```python
from build123d import *

# Parameters (mm, degrees)
SKETCH1_W           = 30
SKETCH1_H           = 70
BOSS_EXTRUDE1_DEPTH = 10.5
SKETCH2_W           = 30
SKETCH2_H           = 35
CUT_EXTRUDE1_DEPTH  = 8
SKETCH3_R           = 3.1
CUT_EXTRUDE2_DEPTH  = 48.2784306
SKETCH4_R           = 1.6
CUT_EXTRUDE3_DEPTH  = 40.5
SKETCH5_W           = 7
SKETCH5_H           = 7
BOSS_EXTRUDE2_DEPTH = 4.5
CUT_EXTRUDE4_REACH  = 76.123
SKETCH6_R           = 1.6


with BuildPart() as part:
    # Sketch1 → Boss-Extrude1 (new body)
    with BuildSketch(Plane(origin=(0, 0, 0), x_dir=(1, 0, 0), z_dir=(0, 1, 0))):
        Rectangle(SKETCH1_W, SKETCH1_H)
    extrude(amount=BOSS_EXTRUDE1_DEPTH)

    # Sketch2 → Cut-Extrude1 (cut)
    with BuildSketch(Plane(origin=(0, 10.5, 0), x_dir=(1, 0, 0), z_dir=(0, 1, 0))):
        Rectangle(SKETCH2_W, SKETCH2_H)
    extrude(amount=-CUT_EXTRUDE1_DEPTH, mode=Mode.SUBTRACT)

    # Sketch3 → Cut-Extrude2 (cut, through all)
    with BuildSketch(Plane(origin=(15, 0, 0), x_dir=(0, 0, -1), z_dir=(1, 0, 0))):
        with Locations((-23, 11.5)):
            Circle(SKETCH3_R)
        with Locations((23, 11.5)):
            Circle(SKETCH3_R)
    extrude(amount=-CUT_EXTRUDE2_DEPTH, mode=Mode.SUBTRACT)

    # Sketch4 → Cut-Extrude3 (cut, through all)
    with BuildSketch(Plane(origin=(0, 10.5, 0), x_dir=(1, 0, 0), z_dir=(0, 1, 0))):
        with Locations(Location((-9.5, -31.5, 0), (0, 0, 270))):
            Circle(SKETCH4_R)
        with Locations(Location((9.5, -31.5, 0), (0, 0, 270))):
            Circle(SKETCH4_R)
        with Locations(Location((-9.5, 28.75, 0), (0, 0, 270))):
            Circle(SKETCH4_R)
        with Locations(Location((9.5, 28.75, 0), (0, 0, 270))):
            Circle(SKETCH4_R)
    extrude(amount=-CUT_EXTRUDE3_DEPTH, mode=Mode.SUBTRACT)

    # Sketch5 → Boss-Extrude2 (add)
    with BuildSketch(Plane(origin=(0, 0, -35), x_dir=(-1, 0, 0), z_dir=(0, 0, -1))):
        with Locations((18.5, 7)):
            Rectangle(SKETCH5_W, SKETCH5_H)
        with Locations((-18.5, 7)):
            Rectangle(SKETCH5_W, SKETCH5_H)
    extrude(amount=-BOSS_EXTRUDE2_DEPTH)

    # Sketch6 → Cut-Extrude4 (cut, up to next)
    with BuildSketch(Plane(origin=(0, 0, -35), x_dir=(-1, 0, 0), z_dir=(0, 0, -1)), mode=Mode.PRIVATE) as cut_extrude4_sk1:
        with Locations((-18.5, 7)):
            Circle(SKETCH6_R)
    cut_extrude4_tool1 = extrude(cut_extrude4_sk1.sketch, amount=-CUT_EXTRUDE4_REACH, mode=Mode.PRIVATE) & part.part
    # Sketch6 → Cut-Extrude4 (cut, up to next)
    with BuildSketch(Plane(origin=(0, 0, -35), x_dir=(-1, 0, 0), z_dir=(0, 0, -1)), mode=Mode.PRIVATE) as cut_extrude4_sk2:
        with Locations((18.5, 7)):
            Circle(SKETCH6_R)
    cut_extrude4_tool2 = extrude(cut_extrude4_sk2.sketch, amount=-CUT_EXTRUDE4_REACH, mode=Mode.PRIVATE) & part.part
    add(cut_extrude4_tool1.solids().sort_by_distance((18.5, 7, -35))[0], mode=Mode.SUBTRACT)
    add(cut_extrude4_tool2.solids().sort_by_distance((-18.5, 7, -35))[0], mode=Mode.SUBTRACT)


solid = part.part
```
Could you check a few things on this model? Use its own coordinates, in mm. A direction names the side the tool comes from. Coordinates: 2 decimals unless noted, no trailing zeros. Loops run counter-clockwise (first coordinate to the right, second up) from the corner with the lowest first, then second, coordinate; pieces in that order, holes last.
1) Imagine slicing it at A-A (x = -18.5). List the corners of the cut face in (y, z) for me, and give its area (3 significant figures).
Reported:
outline: (3.5, -35) - (5.4, -35) - (5.4, -30.5) - (3.5, -30.5) - close; (8.6, -35) - (10.5, -35) - (10.5, -30.5) - (8.6, -30.5) - close
area: 17.1 mm2
2) Please list where these lines run through material, in increasing order: line 1 along X through (y, z) = (2.5, -28.75); line 2 along Y through (x, z) = (-18.5, -32.5); line 3 along Z through (x, y) = (-2, 8).
Reported:
line 1: x = -15 to -11.1, -7.9 to 7.9, 11.1 to 15
line 2: y = 3.5 to 5.4, 8.6 to 10.5
line 3: z = -35 to -17.5, 17.5 to 35
3) Imagine slicing it at B-B (y = 7). List the corners of the cut face in (x, z) for me, and give its area (3 significant figures).
Reported:
outline: (-22, -35) - (-20.1, -35) - (-20.1, -30.5) - (-22, -30.5) - close; (-16.9, -35) - (16.9, -35) - (16.9, -30.5) - (15, -30.5) - (15, -17.5) - (-15, -17.5) - (-15, -30.5) - (-16.9, -30.5) - close; (-15, 17.5) - (15, 17.5) - (15, 35) - (-15, 35) - close; (20.1, -35) - (22, -35) - (22, -30.5) - (20.1, -30.5) - close; hole circle Ø3.2 at (-9.5, -28.75); hole circle Ø3.2 at (-9.5, 31.5); hole circle Ø3.2 at (9.5, -28.75); hole circle Ø3.2 at (9.5, 31.5)
area: 1,050 mm2
4) Imagine slicing it at D-D (y = 1). List the corners of the cut face in (x, z) for me.
Reported:
outline: (-15, -35) - (15, -35) - (15, 35) - (-15, 35) - close; hole circle Ø3.2 at (-9.5, -28.75); hole circle Ø3.2 at (-9.5, 31.5); hole circle Ø3.2 at (9.5, -28.75); hole circle Ø3.2 at (9.5, 31.5)
5) Will these pins go through, and if not, where does the flat tip stop? pin 1 Ø1.3 at (x, z) = (-18, -32) entering from -Y; pin 2 Ø5.5 at (x, y) = (-17, 6) entering from +Z; pin 3 Ø1.9 at (x, z) = (-9.5, 31.5) entering from +Y; pin 4 Ø5 at (y, z) = (9.5, -16) entering from +X.
Reported:
pin 1: stops at y = 3.5
pin 2: stops at z = 35
pin 3: passes through
pin 4: stops at x = 15
6) Which directions (+Z, -Z, +X, -X, +Y, -Y) give clear straight access to the entire face, cutting with the end or side of a thin tool? Please do faces 5 (the face through (19, 9, -30.5)), 6 (the face through (0, 10.5, 30)), 7 (the face through (0, 7, 17.5)).
Reported:
face 5: +Z, +X, +Y, -Y
face 6: +Z, -Z, +X, -X, +Y
face 7: +X, -X, +Y
7) Imagine slicing it at C-C (z = -28.75). List the corners of the cut face in (x, y) for me, and give its area (3 significant figures).
Reported:
outline: (-15, 0) - (-11.1, 0) - (-11.1, 10.5) - (-15, 10.5) - close; (-7.9, 0) - (7.9, 0) - (7.9, 10.5) - (-7.9, 10.5) - close; (11.1, 0) - (15, 0) - (15, 10.5) - (11.1, 10.5) - close
area: 248 mm2
8) Thinking about a two-plate mould opening in X: for faces 1 (the face through (22, 7, -33)), 2 (the face through (8.5, 5.3, -30)), 3 (the face through (-10.5, 5.3, -30)), 4 (the face through (0, 10.5, -19)), which applies, released by +X, released by -X, zero draft, split by the parting line, or undercut?
Reported:
face 1: released by +X
face 2: undercut
face 3: undercut
face 4: zero draft
